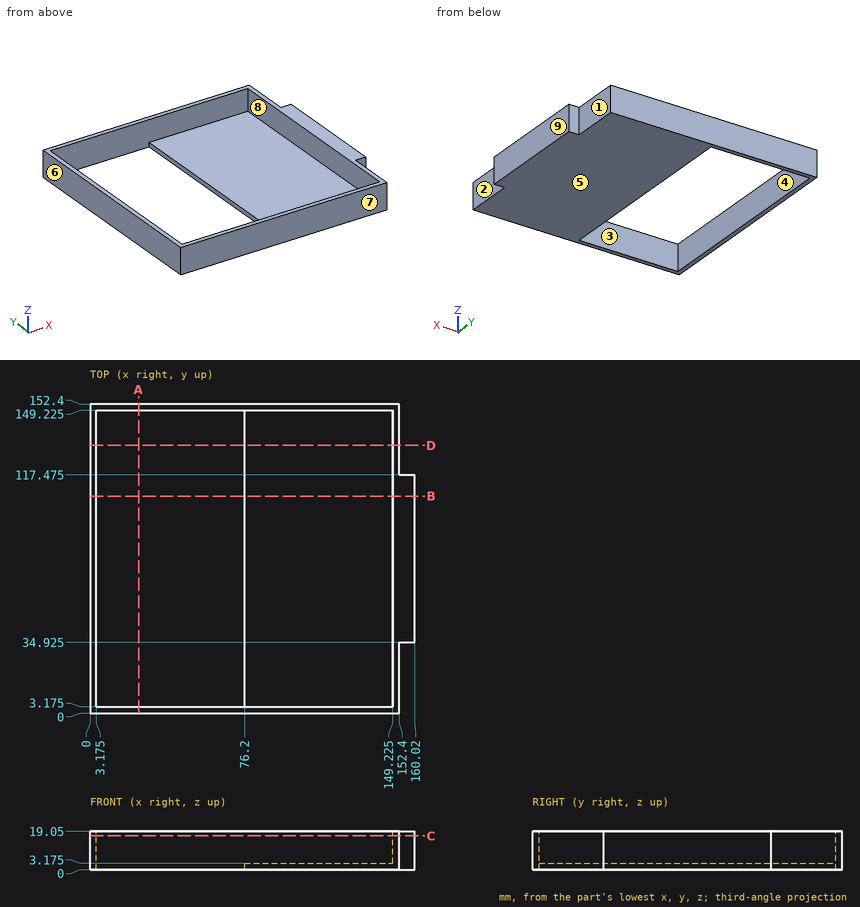
Design review of the part shown in the three views and the two pictorial views. Dimensions are in mm from the part's minimum x, y and z. A direction names the side the tool comes from. Give positions to 0.01 mm unless a question says otherwise; leave off trailing zeros. Loops run counter-clockwise (first coordinate to the right, second up) from the corner with the lowest first, then second, coordinate; pieces in that order, holes last. Notation, with made-up numbers: (67, -36) - (124, -36) arc R23 cw to (124, -21) - close; hole circle Ø2 at (-8, -33). An arc over 180 degrees is marked (long way). Answer as a JSON object with one key per item and string values.
Q1. Mouldability with a two-part tool opening along X and no side actions: class the marked faces 6, 7, 8 and 9 as +X half, -X half, draft (parallel to the pull), parting line (faces both ways), or undercut.
Worked out:
{"face 6": "-X half", "face 7": "draft", "face 8": "undercut", "face 9": "+X half"}
Q2. Insertion check: pin 1 (1 mm diameter, centred on x = 89, y = 34.5, fed in from -Z); pin 2 (6 mm diameter, centred on x = 156.5, z = 7.5, fed in from -Y) (3 decimals); pin 3 (2 mm diameter, centred on y = 121, z = 11.5, fed in from +X); pin 4 (6 mm diameter, centred on x = 155.5, z = 10, fed in from +Y) (3 decimals). Each pin has a flat end and moves straight along its axis. Give the tip position at first contact, or say it passes through.
Worked out:
{"pin 1": "stops at z = 0", "pin 2": "stops at y = 34.925", "pin 3": "stops at x = 152.4", "pin 4": "stops at y = 117.475"}
Q3. For the marked faces 1, 2, 3, 4 and 5, list the 3-axis set-ups (+Z, -Z, +X, -X, +Y, -Y) from which the entire face can be reached by the end or side of a thin tool; tool diameter is ignored.
Worked out:
{"face 1": "+Z, -Z, +X, +Y", "face 2": "+Z, -Z, +X, -Y", "face 3": "+Z", "face 4": "+Z, -Z", "face 5": "-Z, +X, -X, +Y, -Y"}
Q4. Add section D-D on y = 132. State the section outline as (x, z) points (3 decimals), plus the area to 3 significant figures.
Worked out:
{"outline": "(0, 0) - (3.175, 0) - (3.175, 19.05) - (0, 19.05) - close; (76.2, 0) - (152.4, 0) - (152.4, 19.05) - (149.225, 19.05) - (149.225, 3.175) - (76.2, 3.175) - close", "area": "353 mm^2"}
Q5. Add section B-B on y = 107. State the section outline as (x, z) points (3 decimals), plus the area to 3 significant figures.
Worked out:
{"outline": "(0, 0) - (3.175, 0) - (3.175, 19.05) - (0, 19.05) - close; (76.2, 0) - (160.02, 0) - (160.02, 19.05) - (149.225, 19.05) - (149.225, 3.175) - (76.2, 3.175) - close", "area": "498 mm^2"}
Q6. Add section C-C on z = 16.75. State the section outline as (x, y) points (3 decimals), plus the area to 3 significant figures.
Worked out:
{"outline": "(0, 0) - (152.4, 0) - (152.4, 34.925) - (160.02, 34.925) - (160.02, 117.475) - (152.4, 117.475) - (152.4, 152.4) - (0, 152.4) - close; hole (3.175, 3.175) - (149.225, 3.175) - (149.225, 149.225) - (3.175, 149.225) - close", "area": "2,520 mm^2"}
Q7. Add section A-A on x = 24. State the section outline as (y, z) points (3 decimals), plus the area to 3 significant figures.
Worked out:
{"outline": "(0, 0) - (3.175, 0) - (3.175, 19.05) - (0, 19.05) - close; (149.225, 0) - (152.4, 0) - (152.4, 19.05) - (149.225, 19.05) - close", "area": "121 mm^2"}
Q8. To check wall thickness, follow line 1 along Y through (x, z) = (69, 6.5) (3 decimals); line 2 along X through (y, z) = (104, 14.5) (3 decimals). State the ranges of each line that lie inside material, in increasing order.
Worked out:
{"line 1": "y = 0 to 3.175, 149.225 to 152.4", "line 2": "x = 0 to 3.175, 149.225 to 160.02"}
